For this review, take the finished solid that the model builds, in its own axes (mm). A direction names the side the tool comes from. Give positions to 0.01 mm unless a question says otherwise; leave off trailing zeros. Loops run counter-clockwise (first coordinate to the right, second up) from the corner with the lowest first, then second, coordinate; pieces in that order, holes last. Notation, with made-up numbers: (43, 40) - (52, 40) arc R7 ccw to (52, 44) - close; hole circle Ø2 at (78.25, -29.75). An arc over 180 degrees is marked (long way). Answer in a Markdown table with one row per item.
```python
from build123d import *
from build123d.topology import SkipClean

# Parameters (mm, degrees)
SKETCH1_W           = 80
SKETCH1_H           = 80
BOSS_EXTRUDE1_DEPTH = 12.7
SKETCH2_R           = 2
CUT_EXTRUDE1_DEPTH  = 114.847661373
SKETCH3_W           = 60
SKETCH3_H           = 12.7
CUT_EXTRUDE2_DEPTH  = 25
SKETCH4_W           = 60
SKETCH4_H           = 12.7
CUT_EXTRUDE3_DEPTH  = 25
SKETCH5_R           = 2
CUT_EXTRUDE4_DEPTH  = 114.847661373
SKETCH6_W           = 20
SKETCH6_H           = 12.7
CUT_EXTRUDE5_DEPTH  = 20
SKETCH8_W           = 20
SKETCH8_H           = 12.7
CUT_EXTRUDE6_DEPTH  = 20
SKETCH9_W           = 20
SKETCH9_H           = 12.7
SKETCH9_R           = 2
BOSS_EXTRUDE3_DEPTH = 5


with BuildPart() as part:
    # Sketch1 → Boss-Extrude1 (new body)
    with BuildSketch(Plane(origin=(0, 0, 0), x_dir=(1, 0, 0), z_dir=(0, 1, 0))):
        with Locations((-40, 40)):
            Rectangle(SKETCH1_W, SKETCH1_H)
    extrude(amount=BOSS_EXTRUDE1_DEPTH)

    # Sketch2 → Cut-Extrude1 (cut, through all)
    with BuildSketch(Plane.XY):
        with Locations((-75, 6.35)):
            Circle(SKETCH2_R)
        with Locations((-65, 6.35)):
            Circle(SKETCH2_R)
        with Locations((-15, 6.35)):
            Circle(SKETCH2_R)
        with Locations((-5, 6.35)):
            Circle(SKETCH2_R)
    extrude(amount=-CUT_EXTRUDE1_DEPTH, mode=Mode.SUBTRACT)

    # Sketch3 → Cut-Extrude2 (cut)
    with BuildSketch(Plane.XY):
        with Locations((-50, 6.35)):
            Rectangle(SKETCH3_W, SKETCH3_H)
    extrude(amount=-CUT_EXTRUDE2_DEPTH, mode=Mode.SUBTRACT)

    # Sketch4 → Cut-Extrude3 (cut)
    with BuildSketch(Plane(origin=(0, 0, -80), x_dir=(-1, 0, 0), z_dir=(0, 0, -1))):
        with Locations((30, 6.35)):
            Rectangle(SKETCH4_W, SKETCH4_H)
    extrude(amount=-CUT_EXTRUDE3_DEPTH, mode=Mode.SUBTRACT)

    # Sketch5 → Cut-Extrude4 (cut, through all)
    with BuildSketch(Plane(origin=(0, 12.7, 0), x_dir=(1, 0, 0), z_dir=(0, 1, 0))):
        with Locations(Location((-75, 48.65, 0), (0, 0, 270))):
            Circle(SKETCH5_R)
        with Locations(Location((-65, 48.65, 0), (0, 0, 270))):
            Circle(SKETCH5_R)
        with Locations(Location((-75, 31.35, 0), (0, 0, 270))):
            Circle(SKETCH5_R)
        with Locations(Location((-65, 31.35, 0), (0, 0, 270))):
            Circle(SKETCH5_R)
        with Locations(Location((-15, 48.65, 0), (0, 0, 270))):
            Circle(SKETCH5_R)
        with Locations(Location((-5, 48.65, 0), (0, 0, 270))):
            Circle(SKETCH5_R)
        with Locations(Location((-5, 31.35, 0), (0, 0, 270))):
            Circle(SKETCH5_R)
        with Locations(Location((-15, 31.35, 0), (0, 0, 270))):
            Circle(SKETCH5_R)
    extrude(amount=-CUT_EXTRUDE4_DEPTH, mode=Mode.SUBTRACT)

    # Sketch6 → Cut-Extrude5 (cut)
    with BuildSketch(Plane.XY):
        with Locations((-10, 6.35)):
            Rectangle(SKETCH6_W, SKETCH6_H)
    extrude(amount=-CUT_EXTRUDE5_DEPTH, mode=Mode.SUBTRACT)

    # Sketch8 → Cut-Extrude6 (cut)
    with BuildSketch(Plane(origin=(0, 0, -80), x_dir=(-1, 0, 0), z_dir=(0, 0, -1))):
        with Locations((70, 6.35)):
            Rectangle(SKETCH8_W, SKETCH8_H)
    extrude(amount=-CUT_EXTRUDE6_DEPTH, mode=Mode.SUBTRACT)

    # Sketch9 → Boss-Extrude3 (add)
    # profile 1 of 2: a face of its own
    with SkipClean():  # the faces are left unmerged after this step: merging them gives an invalid solid
        with BuildSketch(Plane.XZ):
            with Locations((-10, -48.65)):
                Rectangle(SKETCH9_W, SKETCH9_H)
            with Locations((-15, -48.65)):
                Circle(SKETCH9_R, mode=Mode.SUBTRACT)
            with Locations((-5, -48.65)):
                Circle(SKETCH9_R, mode=Mode.SUBTRACT)
        # profile 2 of 2: a face of its own
        with BuildSketch(Plane.XZ):
            with Locations((-70, -31.35)):
                Rectangle(SKETCH9_W, SKETCH9_H)
            with Locations((-65, -31.35)):
                Circle(SKETCH9_R, mode=Mode.SUBTRACT)
            with Locations((-75, -31.35)):
                Circle(SKETCH9_R, mode=Mode.SUBTRACT)
        extrude(amount=BOSS_EXTRUDE3_DEPTH)


solid = part.part
```
1. We need section A-A, the plane y = -4. Give the boundary of the cut face in (x, z).
Values:
| item | result |
|---|---|
| outline | (-80, -37.7) - (-60, -37.7) - (-60, -25) - (-80, -25) - close; (-20, -55) - (0, -55) - (0, -42.3) - (-20, -42.3) - close; hole circle Ø4 at (-75, -31.35); hole circle Ø4 at (-65, -31.35); hole circle Ø4 at (-15, -48.65); hole circle Ø4 at (-5, -48.65) |
2. Mouldability with a two-part tool opening along X and no side actions: class faces 4 (the face through (-41, 12.7, -40)), 5 (the face through (-20, 6, -22)), 6 (the face through (-77, 6.4, -55.5)), 7 (the face through (-4.912, 2.514, -33.348)) as released by +X, released by -X, zero draft, split by the parting line, or undercut.
Values:
| item | result |
|---|---|
| face 4 | zero draft |
| face 5 | released by -X |
| face 6 | undercut |
| face 7 | undercut |
3. Wall thickness on line 1 (X direction, y = -3.6, z = -48.65); line 2 (Z direction, x = -15, y = 1.5); line 3 (X direction, y = 4.25, z = -48.65): over which ranges is each line inside the solid? List them lowest first. Write a range as [from, to].
Values:
| item | result |
|---|---|
| line 1 | x = [-20, -17], [-13, -7], [-3, 0] |
| line 2 | z = [-55, -50.65], [-46.65, -33.35], [-29.35, -20] |
| line 3 | x = [-80, -77], [-73, -67], [-63, -17], [-13, -7], [-3, 0] |
4. For faces 1 (the face through (-41, 0, -40)), 2 (the face through (-10, -2, -42.3)), 3 (the face through (-67, 6.4, -55.5)), list the 3-axis set-ups (+Z, -Z, +X, -X, +Y, -Y) from which the entire face can be reached by the end or side of a thin tool; tool diameter is ignored.
Values:
| item | result |
|---|---|
| face 1 | -Y |
| face 2 | +Z, +X, -X, -Y |
| face 3 | +Z, -Z |
5. Clearance check with flat-ended pins moving along their axes: pin 1 (5 mm diameter, centred on x = -15, z = -31.35, fed in from -Y); pin 2 (5 mm diameter, centred on x = -15, z = -48.65, fed in from -Y); pin 3 (1.5 mm diameter, centred on x = -33.5, y = 8.5, fed in from -Z); pin 4 (4 mm diameter, centred on x = -46, y = 5, fed in from +Z). State where each tip first meets the part, or that it passes through.
Values:
| item | result |
|---|---|
| pin 1 | stops at y = 0 |
| pin 2 | stops at y = -5 |
| pin 3 | stops at z = -55 |
| pin 4 | stops at z = -25 |
6. We need section C-C, the plane z = -45. Give the boundary of the cut face in (x, y), and give its area (3 significant figures).
Values:
| item | result |
|---|---|
| outline | (-80, 0) - (-20, 0) - (-20, -5) - (0, -5) - (0, 12.7) - (-80, 12.7) - close; hole circle Ø4 at (-75, 6.35); hole circle Ø4 at (-65, 6.35); hole circle Ø4 at (-15, 6.35); hole circle Ø4 at (-5, 6.35) |
| area | 1,070 mm^2 |
7. We need section B-B, the plane x = -75. Give the boundary of the cut face in (y, z).
Values:
| item | result |
|---|---|
| outline | (-5, -37.7) - (0, -37.7) - (0, -46.65) - (4.35, -46.65) - (4.35, -33.35) - (-5, -33.35) - close; (-5, -29.35) - (4.35, -29.35) - (4.35, -25) - (-5, -25) - close; (0, -60) - (4.35, -60) - (4.35, -50.65) - (0, -50.65) - close; (8.35, -60) - (12.7, -60) - (12.7, -50.65) - (8.35, -50.65) - close; (8.35, -46.65) - (12.7, -46.65) - (12.7, -33.35) - (8.35, -33.35) - close; (8.35, -29.35) - (12.7, -29.35) - (12.7, -25) - (8.35, -25) - close |
